Could you check a few things on this model? Use its own coordinates, in mm. Face numbers are marked on the shaded views. A direction names the side the tool comes from. Round coordinates to 2 decimals unless told otherwise and drop trailing zeros. Loops run counter-clockwise (first coordinate to the right, second up) from the corner with the lowest first, then second, coordinate; pieces in that order, holes last. Notation, with made-up numbers: (32.25, -21.75) - (60.25, -21.75) arc R25 ccw to (60.25, 2.25) - close; hole circle Ø2 at (76, 4). An arc over 180 degrees is marked (long way). Use one line per item in the form item = value.
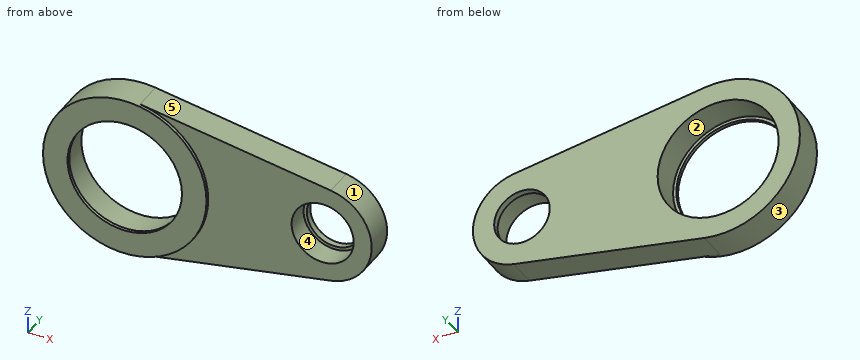
```python
from build123d import *

# Parameters (mm, degrees)
SKETCH_1_R           = 25
SKETCH_1_R_2         = 17.5
EXTRUDE_1_DEPTH      = 5
SKETCH_2_R           = 25
SKETCH_2_R_2         = 18.5
EXTRUDE_2_DEPTH      = 5
EXTRUDE_3_DEPTH      = 9
SKETCH_7_R           = 18.5
CUT_EXTRUDE_4_DEPTH  = 4
SKETCH_13_R          = 9.5
CUT_EXTRUDE_9_DEPTH  = 7
SKETCH_14_R          = 8.5
CUT_EXTRUDE_10_DEPTH = 3


with BuildPart() as part:
    # 스케치1 → 보스-돌출1 (new body)
    with BuildSketch(Plane(origin=(0, 0, 0), x_dir=(1, 0, 0), z_dir=(0, 1, 0))):
        Circle(SKETCH_1_R)
        Circle(SKETCH_1_R_2, mode=Mode.SUBTRACT)
    extrude(amount=EXTRUDE_1_DEPTH)

    # 스케치2 → 보스-돌출2 (add)
    with BuildSketch(Plane(origin=(0, 5, 0), x_dir=(1, 0, 0), z_dir=(0, 1, 0))):
        Circle(SKETCH_2_R)
        Circle(SKETCH_2_R_2, mode=Mode.SUBTRACT)
    extrude(amount=EXTRUDE_2_DEPTH)

    # 스케치3 → 보스-돌출3 (add)
    with BuildSketch(Plane(origin=(0, 10, 0), x_dir=(1, 0, 0), z_dir=(0, 1, 0))):
        with BuildLine():
            Line((4.166666667, 24.65033243), (62.5, 14.790199458))
            ThreePointArc((62.5, 14.790199458), (75, 0), (62.5, -14.790199458))
            Line((62.5, -14.790199458), (4.166666667, -24.65033243))
            ThreePointArc((4.166666667, -24.65033243), (25, 0), (4.166666667, 24.65033243))
        make_face()
    extrude(amount=-EXTRUDE_3_DEPTH)

    # 스케치7 → 컷-돌출4 (cut)
    with BuildSketch(Plane(origin=(0, 5, 0), x_dir=(1, 0, 0), z_dir=(0, 1, 0))):
        Circle(SKETCH_7_R)
    extrude(amount=-CUT_EXTRUDE_4_DEPTH, mode=Mode.SUBTRACT)

    # 스케치13 → 컷-돌출9 (cut)
    with BuildSketch(Plane.XZ.offset(-1)):
        with Locations((60, 0)):
            Circle(SKETCH_13_R)
    extrude(amount=-CUT_EXTRUDE_9_DEPTH, mode=Mode.SUBTRACT)

    # 스케치14 → 컷-돌출10 (cut, through all)
    with BuildSketch(Plane.XZ.offset(-8)):
        with Locations((60, 0)):
            Circle(SKETCH_14_R)
    extrude(amount=-CUT_EXTRUDE_10_DEPTH, mode=Mode.SUBTRACT)


solid = part.part
```
1. If we section it at C-C, the plane y = 5.75: Write out the boundary of the cut face in (x, z), plus the area to 3 significant figures.
Solution:
outline = (4.17, -24.65) - (62.5, -14.79) arc R15 ccw to (62.5, 14.79) - (4.17, 24.65) arc R25 ccw (long way) to start; hole circle Ø37 at (0, 0); hole circle Ø19 at (60, 0)
area = 2,410 mm^2
2. On a 3-axis mill with a long thin cutter (end or side, diameter ignored), from which of +Z, -Z, +X, -X, +Y, -Y can I reach the whole of each face in a straight line? I mean the marked faces 1 and 2. Say none if no direction works.
Solution:
face_1 = +X, +Y, -Y
face_2 = +Y
3. Please list where these lines run through material, in increasing order: line 1 along Z through (x, y) = (0, 5.5); line 2 along X through (y, z) = (8.5, -5.5); line 3 along Y through (x, z) = (52, -8).
Solution:
line_1 = -25 to -18.5, 18.5 to 25
line_2 = -24.39 to -17.66, 17.66 to 53.52, 66.48 to 73.96
line_3 = 1 to 10
4. If we section it at D-D, the plane x = 60: Write out the boundary of the cut face in (y, z), plus the area to 3 significant figures.
Solution:
outline = (1, -15.21) - (10, -15.21) - (10, -8.5) - (8, -8.5) - (8, -9.5) - (1, -9.5) - close; (1, 9.5) - (8, 9.5) - (8, 8.5) - (10, 8.5) - (10, 15.21) - (1, 15.21) - close
area = 107 mm^2
5. If we section it at A-A, the plane z = 0: Write out the boundary of the cut face in (x, y).
Solution:
outline = (-25, 0) - (-17.5, 0) - (-17.5, 1) - (-18.5, 1) - (-18.5, 10) - (-25, 10) - close; (17.5, 0) - (25, 0) - (25, 1) - (50.5, 1) - (50.5, 8) - (51.5, 8) - (51.5, 10) - (18.5, 10) - (18.5, 1) - (17.5, 1) - close; (68.5, 8) - (69.5, 8) - (69.5, 1) - (75, 1) - (75, 10) - (68.5, 10) - close
6. If we section it at B-B, the plane x = 0: Write out the boundary of the cut face in (y, z).
Solution:
outline = (0, -25) - (10, -25) - (10, -18.5) - (1, -18.5) - (1, -17.5) - (0, -17.5) - close; (0, 17.5) - (1, 17.5) - (1, 18.5) - (10, 18.5) - (10, 25) - (0, 25) - close
7. We'd pull the mould along Z, two halves only. Please class the marked faces 3, 4 and 5: +Z half, -Z half, draft (parallel to the pull), parting line (faces both ways), or undercut.
Solution:
face_3 = parting line
face_4 = undercut
face_5 = +Z half
8. For P1, Ø1, axis at y = 7, z = -5.5, coming from the -X side; P2, Ø4, axis at y = 2, z = -9, coming from the -X side; P3, Ø2, axis at y = 6.5, z = -12, coming from the -X side; P4, Ø4, axis at x = 4, z = 16.5, coming from the -Y side, each with a flat end and sliding along its axis, tell me the tip position at first contact or that it passes through.
Solution:
P1 = -24.49
P2 = -24
P3 = -22.45
P4 = 0
